Check sheet for the modelled part. Datum: model origin and axes. Units: mm. A direction names the side the tool comes from. Give positions to 0.01 mm unless a question says otherwise; leave off trailing zeros. Loops run counter-clockwise (first coordinate to the right, second up) from the corner with the lowest first, then second, coordinate; pieces in that order, holes last. Notation, with made-up numbers: (27.25, 31) -> (40.25, 31) arc R21 cw to (40.25, 68) -> close; hole circle Ø11 at (20, 84). An arc over 180 degrees is marked (long way). Write each question's results on one line, items separated by ' | '. Start each with the question number.
Item 1: Cross-section at B-B on z = 36.5. Enter the section's corners in (x, y).
Item 2: Access from +Z, -Z, +X, -X, +Y, -Y to the whole of each face (thin tool, end or side, straight path). Record for faces 5 (the face through (47, 0, 85)), 6 (the face through (35, 0, 10)), 7 (the face through (-20, 0, 10)).
Item 3: Cross-section at C-C on x = -35. Enter the section's corners in (y, z), then the cut area to 3 significant figures.
Item 4: Gauge pin test, flat ends, axial feed: pin 1 Ø5.5 at (x, y) = (47.5, 3) entering from +Z; pin 2 Ø5 at (y, z) = (1, 44.5) entering from -X; pin 3 Ø5 at (x, y) = (36.5, -0.5) entering from +Z; pin 4 Ø1 at (y, z) = (2.5, 85) entering from -X. Record the tip position at first contact, or that the pin passes through.
Item 5: Cross-section at D-D on z = 100. Enter the section's corners in (x, y), then the cut area to 3 significant figures.
Item 6: Cross-section at A-A on z = 14. Enter the section's corners in (x, y).
Item 7: Mould release check, pull along Z, two halves, no side actions. Record for faces 1 (the face through (35, 0, 20)), 2 (the face through (12, -5, 9)), 3 (the face through (-1, 0, 0)), 4 (the face through (46, -4, 55)): pulls with the +Z half, pulls with the -Z half, needs draft (parallel to the pull), parting line crosses it, or undercut.
Item 8: Scan lines: line 1 along Z through (x, y) = (30, -0.5); line 2 along X through (y, z) = (-1.5, 26.5); line 3 along X through (y, z) = (2, 51.5). Record each from-to range of solid material in increasing order.
from build123d import *

# Parameters (mm, degrees)
F0_W      = 110
F0_H      = 10
F1_DEPTH  = 10
F2_W      = 10
F2_H      = 10
F3_DEPTH  = 45
F4_R      = 3
F5_DEPTH  = 54
F12_DEPTH = 10


with BuildPart() as f1:
    # F0 (on Top) → F1 (new body)
    with BuildSketch(Plane.XY):
        Rectangle(F0_W, F0_H)
    extrude(amount=F1_DEPTH)

    # F2 (on face) → F3 (join)
    with BuildSketch(Plane.XY.offset(10)):
        with Locations((50, 0)):
            Rectangle(F2_W, F2_H)
    extrude(amount=F3_DEPTH)

    # F4 (on face) → F5 (join)
    with BuildSketch(Plane.XY.offset(55)):
        with Locations((50, 0)):
            Circle(F4_R)
    extrude(amount=F5_DEPTH)

    # F7 (on mid) → F9 (revolve)
    with BuildSketch(Plane(origin=(50, 0, 0), x_dir=(0, -1, 0), z_dir=(-1, 0, 0))):
        Polygon((0, 70), (0, 55), (5, 55), align=None)
    revolve(axis=Axis((50, 0, 50.9786196053), (0, 0, 1)))

    # F11 (on offset) → F12 (join, through all)
    with BuildSketch(Plane(origin=(0, 5, 0), x_dir=(-1, 0, 0), z_dir=(0, 1, 0))):
        Polygon((-25, 10), (-15, 10), (-45, 40), (-45, 30), align=None)
    extrude(amount=-F12_DEPTH)


solid = f1.part
Answer sheet:
1) outline: (41.5, -5) -> (55, -5) -> (55, 5) -> (41.5, 5) -> close
2) face 5: +Z | face 6: +Y, -Y | face 7: +Z, -X, +Y, -Y
3) outline: (-5, 0) -> (5, 0) -> (5, 10) -> (-5, 10) -> close | area: 100 mm²
4) pin 1: stops at z = 109 | pin 2: stops at x = 45 | pin 3: stops at z = 34 | pin 4: stops at x = 47.76
5) outline: circle Ø6 at (50, 0) | area: 28.3 mm²
6) outline: (19, -5) -> (29, -5) -> (29, 5) -> (19, 5) -> close; (45, -5) -> (55, -5) -> (55, 5) -> (45, 5) -> close
7) face 1: undercut | face 2: needs draft | face 3: pulls with the -Z half | face 4: pulls with the +Z half
8) line 1: z = 0 to 10, 15 to 25 | line 2: x = 31.5 to 41.5, 45 to 55 | line 3: x = 45 to 55
